Source: CAD feature listing. Evaluate the final solid. Frame: model axes, mm. A direction names the side the tool comes from. Give positions to 0.01 mm unless a question says otherwise; leave off trailing zeros. Order: outer loops, then holes, each group sorted by start corner. A loop starts at its lowest first (then second) coordinate and runs counter-clockwise, first axis right, second up.
```python
from build123d import *

# Parameters (mm, degrees)
SKETCH1_W                                 = 76.2
SKETCH1_H                                 = 39.6875
BASE_DEPTH                                = 6.35
SKETCH2_W                                 = 76.2
SKETCH2_H                                 = 6.35
WALLS_DEPTH                               = 25.4
SCREW_START                               = -39.6875
SCREW_HOLE_OUTLINE_R                      = 2.77876
SCREW_HOLE_DEPTH                          = 39.6875
HOLE_PATTERN_COUNT                        = 2
HOLE_PATTERN_PITCH                        = 25.4
TOP_SECTION_DEPTH                         = 76.2
BOLT_HOLE_CHAMFER_SIZE                    = 15.24
BOLT_HOLE_CHAMFER_SIZE2                   = 41.871555872
SKETCH24_R                                = 12.7
TEMP_POLE_HOLE_DEPTH                      = 76.2
SKETCH26_R                                = 3.96875
TEMP_BOLT_HOLES_DEPTH                     = 138.966445762
TOP_SECTION_BROOM_SUPPORT_HOLE_DEPTH      = 115.222803793
TOP_SECTION_BROOM_SUPPORT_HOLE_DEPTH_BACK = 115.222803793
SKETCH28_R                                = 3.175


# Read off the part's stored shape, not the designer's step: Screw hole
with BuildPart() as part:
    # Sketch1 → Base (new body)
    with BuildSketch(Plane(origin=(0, 0, 0), x_dir=(1, 0, 0), z_dir=(0, 1, 0))):
        with Locations((38.1, 19.84375)):
            Rectangle(SKETCH1_W, SKETCH1_H)
    extrude(amount=BASE_DEPTH)

    # Sketch2 → Walls (add)
    with BuildSketch(Plane.XZ):
        with Locations((38.1, -3.175)):
            Rectangle(SKETCH2_W, SKETCH2_H)
        with Locations((38.1, -36.5125)):
            Rectangle(SKETCH2_W, SKETCH2_H)
    extrude(amount=WALLS_DEPTH)

    # Screw hole outline → Screw hole (cut)
    with BuildSketch(Plane.XY.offset(SCREW_START)):
        with Locations((50.8, -9.525)):
            Circle(SCREW_HOLE_OUTLINE_R)
    screw_hole = extrude(amount=SCREW_HOLE_DEPTH, mode=Mode.SUBTRACT)

    # Hole pattern: Screw hole ×2
    with Locations(*[(-i * HOLE_PATTERN_PITCH, 0, 0) for i in range(1, HOLE_PATTERN_COUNT)]):
        add(screw_hole, mode=Mode.SUBTRACT)

    # Sketch7 → Top section (add)
    with BuildSketch(Plane(origin=(0, 6.35, 0), x_dir=(1, 0, 0), z_dir=(0, 1, 0))):
        with BuildLine():
            Line((4.766372527, 30.00375), (4.766372527, 9.68375))
            Line((4.766372527, 9.68375), (25.086372527, 9.68375))
            ThreePointArc((25.086372527, 9.68375), (21.59, 19.84375), (25.086372527, 30.00375))
            Line((25.086372527, 30.00375), (4.766372527, 30.00375))
        make_face()
        with BuildLine():
            ThreePointArc((25.086372527, 30.00375), (21.59, 19.84375), (25.086372527, 9.68375))
            Line((25.086372527, 9.68375), (25.086372527, 30.00375))
        make_face()
        with BuildLine():
            Line((25.086372527, 30.00375), (25.086372527, 9.68375))
            ThreePointArc((25.086372527, 9.68375), (38.1, 3.33375), (51.113627473, 9.68375))
            Line((51.113627473, 9.68375), (51.113627473, 30.00375))
            ThreePointArc((51.113627473, 30.00375), (38.1, 36.35375), (25.086372527, 30.00375))
        make_face()
        with BuildLine():
            Line((51.113627473, 30.00375), (51.113627473, 9.68375))
            ThreePointArc((51.113627473, 9.68375), (53.711455563, 14.471361778), (54.61, 19.84375))
            ThreePointArc((54.61, 19.84375), (53.711455563, 25.216138222), (51.113627473, 30.00375))
        make_face()
        with BuildLine():
            ThreePointArc((54.61, 19.84375), (53.711455563, 14.471361778), (51.113627473, 9.68375))
            Line((51.113627473, 9.68375), (71.433627473, 9.68375))
            Line((71.433627473, 9.68375), (71.433627473, 30.00375))
            Line((71.433627473, 30.00375), (51.113627473, 30.00375))
            ThreePointArc((51.113627473, 30.00375), (53.711455563, 25.216138222), (54.61, 19.84375))
        make_face()
    extrude(amount=TOP_SECTION_DEPTH)

    # Bolt hole chamfer
    bolt_hole_chamfer_edges = [part.edges().sort_by_distance(p)[0] for p in [
        (4.766372527, 82.55, -19.84375),
        (71.433627473, 82.55, -19.84375),
    ]]
    bolt_hole_chamfer_side = [part.faces().sort_by_distance(p)[0] for p in [
        (38.1, 82.55, -19.84375),
    ]]
    chamfer(bolt_hole_chamfer_edges, length=BOLT_HOLE_CHAMFER_SIZE, length2=BOLT_HOLE_CHAMFER_SIZE2, reference=bolt_hole_chamfer_side[0])

    # Sketch24 → Temp Pole Hole (cut)
    with BuildSketch(Plane(origin=(0, 82.55, 0), x_dir=(1, 0, 0), z_dir=(0, 1, 0))):
        with Locations(Location((38.1, 19.84375, 0), (0, 0, 270))):
            Circle(SKETCH24_R)
    extrude(amount=-TEMP_POLE_HOLE_DEPTH, mode=Mode.SUBTRACT)

    # Sketch26 → Temp bolt holes (cut, through all)
    with BuildSketch(Plane(origin=(0, 82.55, 0), x_dir=(1, 0, 0), z_dir=(0, 1, 0))):
        with Locations((12.7, 19.84375)):
            Circle(SKETCH26_R)
    temp_bolt_holes = extrude(amount=-TEMP_BOLT_HOLES_DEPTH, mode=Mode.SUBTRACT)

    # Temp bolt hole mirror: Temp bolt holes across plane
    add(temp_bolt_holes.mirror(Plane(origin=(38.1, 0, 0), x_dir=(0, 0, 1), z_dir=(1, 0, 0))), mode=Mode.SUBTRACT)

    # Sketch28 → Top section broom support hole (cut, two sides: drawn at the far end of the back side and taken through both)
    with BuildSketch(Plane.XY.offset(-19.05).offset(-TOP_SECTION_BROOM_SUPPORT_HOLE_DEPTH_BACK)):
        with Locations((38.1, 44.45)):
            Circle(SKETCH28_R)
    extrude(amount=TOP_SECTION_BROOM_SUPPORT_HOLE_DEPTH + TOP_SECTION_BROOM_SUPPORT_HOLE_DEPTH_BACK, mode=Mode.SUBTRACT)


solid = part.part
```
1) Draft query along Y for faces 1 (the flat face through (21, 6.35, -33)), 2 (the cylindrical face through (28.05, -8.69, -36.56)), 3 (the flat face through (38, -13, -6.35)). Return one class per face: +Y half, -Y half, draft (parallel to the pull), parting line (faces both ways), or undercut.
Report:
face 1: +Y half
face 2: undercut
face 3: draft
2) Reachability of faces 4 (the flat face through (38, -13, -33.338)), 5 (the flat face through (4.766, 23, -20)), 6 (the cylindrical face through (41.614, 43.917, -35.975)), 7 (the cylindrical face through (41.91, 44.98, -7.73)), 8 (the flat face through (17, 35, -30.004)) from +Z, -Z, +X, -X, +Y, -Y: full face, straight path, thin tool, end or side. Return the list, or none.
Report:
face 4: +X, -X, -Y
face 5: +Z, -Z, -X, +Y
face 6: -Z, +Y
face 7: +Y
face 8: -Z, -X, +Y
3) Pin query (flat end, axial travel): pin 1 (1 mm diameter, centred on x = 38, z = -26, fed in from -Y); pin 2 (9 mm diameter, centred on x = 25.4, y = -9.525, fed in from +Z); pin 3 (16.5 mm diameter, centred on x = 15.5, y = 53.5, fed in from -Z); pin 4 (10 mm diameter, centred on x = 38.1, y = 44.45, fed in from -Z). Return the tip coordinate at first contact, or that it passes through.
Report:
pin 1: stops at y = 0
pin 2: stops at z = 0
pin 3: stops at z = -30
pin 4: stops at z = -36.35
4) Material intervals for L1, parallel to Z at x = 59.5, y = -10; L2, parallel to X at y = 28, z = -20; L3, parallel to Y at x = 38.1, z = -6.7 (3 decimals), sorted ascending.
Report:
L1: z = -39.69 to -33.34, -6.35 to 0
L2: x = 4.77 to 8.73, 16.67 to 25.4, 50.8 to 59.53, 67.47 to 71.43
L3: y = 0 to 41.275, 47.625 to 82.55
5) Section query B-B, the plane y = -17. Return the cut outline in (x, z).
Report:
outline: (0, -39.69) - (76.2, -39.69) - (76.2, -33.34) - (0, -33.34) - close; (0, -6.35) - (76.2, -6.35) - (76.2, 0) - (0, 0) - close
6) Section query C-C, the plane y = 44.45. Return the cut outline in (x, z) (1 decimal), and give its area (3 significant figures).
Report:
outline: (6.1, -30) - (25.1, -30) arc R16.5 ccw to (34.9, -36) - (34.9, -32.1) arc R12.7 cw to (34.9, -7.5) - (34.9, -3.6) arc R16.5 ccw to (25.1, -9.7) - (6.1, -9.7) - close; (41.3, -36) arc R16.5 ccw to (51.1, -30) - (70.1, -30) - (70.1, -9.7) - (51.1, -9.7) arc R16.5 ccw to (41.3, -3.6) - (41.3, -7.5) arc R12.7 cw to (41.3, -32.1) - close; hole circle Ø7.9 at (12.7, -19.8); hole circle Ø7.9 at (63.5, -19.8)
area: 875 mm2
7) Section query A-A, the plane x = 38.1. Count the separate pieces of the cut face and the enclosed holes in it, and give its area (3 significant figures).
Report:
separate pieces: 3
enclosed holes: 0
area: 1,110 mm2
